Can you work these out from the model? Positions are in its coordinate system, mm. Round coordinates to 2 decimals unless told otherwise and drop trailing zeros. Loops run counter-clockwise (first coordinate to the right, second up) from the corner with the lowest first, then second, coordinate; pieces in that order, holes last. Notation, with made-up numbers: M -2.5,74.5 L 37.5,74.5 A21 ccw 37.5,87.5 Z; hole C 70.25,22 d8. An arc over 180 degrees is marked long. Return JSON: item names as keys, results as strings.
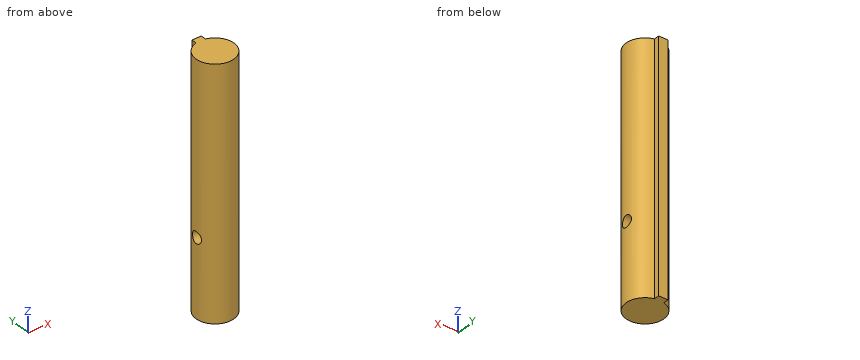
```python
from build123d import *

# Parameters (mm, degrees)
BOSS_EXTRUDE1_DEPTH = 52
SKETCH2_R           = 1.225
CUT_EXTRUDE1_DEPTH  = 25


with BuildPart() as part:
    # Sketch1 → Boss-Extrude1 (new body)
    with BuildSketch(Plane.XY):
        with BuildLine():
            Line((-1, 3.872983346), (-1, 5.002983346))
            Line((-1, 5.002983346), (1, 5.002983346))
            Line((1, 5.002983346), (1, 3.872983346))
            ThreePointArc((1, 3.872983346), (0, -4), (-1, 3.872983346))
        make_face()
    extrude(amount=BOSS_EXTRUDE1_DEPTH)

    # Sketch2 → Cut-Extrude1 (cut, symmetric)
    with BuildSketch(Plane(origin=(0, 0, 0), x_dir=(0, 0, -1), z_dir=(1, 0, 0))):
        with Locations((-16.3, 0)):
            Circle(SKETCH2_R)
    extrude(amount=CUT_EXTRUDE1_DEPTH, both=True, mode=Mode.SUBTRACT)


solid = part.part
```
Q1. Suppose I cut it at B-B, the plane x = -1.75. Please give me the cut outline in (y, z) (3 decimals).
Results:
{"outline": "M -3.597,0 L 3.597,0 L 3.597,52 L -3.597,52 Z; hole C 0,16.3 d2.45"}
Q2. Suppose I cut it at C-C, the plane z = 16.3. Please give me the cut outline in (x, y) (3 decimals).
Results:
{"outline": "M -3.808,-1.225 A4 ccw 3.808,-1.225 Z; M -3.808,1.225 L 3.808,1.225 A4 ccw 1,3.873 L 1,5.003 L -1,5.003 L -1,3.873 A4 ccw Z"}
Q3. Suppose I cut it at A-A, the plane y = 0. Please give me the cut outline in (x, z) (3 decimals), plus the area to 3 significant figures.
Results:
{"outline": "M -4,0 L 4,0 L 4,15.075 L -4,15.075 Z; M -4,17.525 L 4,17.525 L 4,52 L -4,52 Z", "area": "396 mm2"}
Q4. Suppose I cut it at D-D, the plane z = 11. Please give me the cut outline in (x, y), plus the area to 3 significant figures.
Results:
{"outline": "M -1,3.87 A4 ccw long 1,3.87 L 1,5 L -1,5 Z", "area": "52.4 mm2"}
Q5. I'm going to push flat-ended pins straight in: pin 1 Ø0.6 at (y, z) = (4, 32.5) entering from -X; pin 2 Ø0.9 at (y, z) = (4.5, 25) entering from +X; pin 3 Ø1.5 at (y, z) = (0, 16.3) entering from +X. Where does each tip first touch, or does it pass through?
Results:
{"pin 1": "stops at x = -1.52", "pin 2": "stops at x = 1", "pin 3": "passes through"}
Q6. If I drill on line 1 along Z through (x, y) = (-1.5, 0) (3 decimals); line 2 along Y through (x, z) = (0.25, 16.3) (3 decimals); line 3 along Y through (x, z) = (0.25, 50), over which ranges is the centre line in solid material (lowest first)?
Results:
{"line 1": "z = 0 to 15.075, 17.525 to 52", "line 2": "y = -3.992 to -1.225, 1.225 to 5.003", "line 3": "y = -3.99 to 5"}
